Geometry: final body of the model. Coordinates: model frame, mm. A direction names the side the tool comes from. Coordinates: 2 decimals unless noted, no trailing zeros. Use CSV: the item, a comma, the result in double quotes. Start each with the question number.
from build123d import *

# Parameters (mm, degrees)
SKETCH1_R           = 1.5875
BOSS_EXTRUDE1_DEPTH = 1.5748
SKETCH2_W           = 5.842
SKETCH2_H           = 5.842
CUT_EXTRUDE1_DEPTH  = 0.0254
CUT_EXTRUDE2_START  = -1.5748
SKETCH2_2_W         = 5.842
SKETCH2_2_H         = 5.842
CUT_EXTRUDE2_DEPTH  = 0.0254


with BuildPart() as part:
    # Sketch1 → Boss-Extrude1 (new body)
    with BuildSketch(Plane(origin=(0, 0, 0), x_dir=(1, 0, 0), z_dir=(0, 1, 0))):
        Polygon((85.774022, 22.698964), (85.774022, 12.099036), (86.36, 11.557), (86.36, 0), (0, 0), (0, 54.61), (86.36, 54.61), (86.36, 23.241), align=None)
        with Locations((3.175, 51.435)):
            Circle(SKETCH1_R, mode=Mode.SUBTRACT)
        with Locations((3.175, 3.175)):
            Circle(SKETCH1_R, mode=Mode.SUBTRACT)
        with Locations((83.185, 3.175)):
            Circle(SKETCH1_R, mode=Mode.SUBTRACT)
        with Locations((83.185, 51.435)):
            Circle(SKETCH1_R, mode=Mode.SUBTRACT)
    extrude(amount=BOSS_EXTRUDE1_DEPTH)

    # Sketch2 → Cut-Extrude1 (cut)
    with BuildSketch(Plane(origin=(0, 1.5748, 0), x_dir=(1, 0, 0), z_dir=(0, 1, 0))):
        with Locations((3.175, 51.435)):
            Rectangle(SKETCH2_W, SKETCH2_H)
        with Locations((3.175, 3.175)):
            Rectangle(SKETCH2_W, SKETCH2_H)
        with Locations((83.185, 3.175)):
            Rectangle(SKETCH2_W, SKETCH2_H)
        with Locations((83.185, 51.435)):
            Rectangle(SKETCH2_W, SKETCH2_H)
    extrude(amount=-CUT_EXTRUDE1_DEPTH, mode=Mode.SUBTRACT)

    # Sketch2<2> → Cut-Extrude2 (cut)
    with BuildSketch(Plane(origin=(0, 1.5748, 0), x_dir=(1, 0, 0), z_dir=(0, 1, 0)).offset(CUT_EXTRUDE2_START)):
        with Locations((3.175, 51.435)):
            Rectangle(SKETCH2_2_W, SKETCH2_2_H)
        with Locations((3.175, 3.175)):
            Rectangle(SKETCH2_2_W, SKETCH2_2_H)
        with Locations((83.185, 3.175)):
            Rectangle(SKETCH2_2_W, SKETCH2_2_H)
        with Locations((83.185, 51.435)):
            Rectangle(SKETCH2_2_W, SKETCH2_2_H)
    extrude(amount=CUT_EXTRUDE2_DEPTH, mode=Mode.SUBTRACT)


solid = part.part
(1) Mould query, pull axis X, two halves, no side actions, for faces 3 (the face through (84.038, 0.777, -4.514)), 4 (the face through (2.005, 0.777, -4.248)), 5 (the face through (86.36, 1, -6)). Classes: pulls with the +X half, pulls with the -X half, needs draft (parallel to the pull), parting line crosses it, or undercut.
(2) First-contact query: pin 1 (3 mm diameter, centred on x = 2.5, z = -2.5, fed in from -Y); pin 2 (3 mm diameter, centred on x = 82, z = -4.5, fed in from +Y). Flat tips, straight axial feed; report the tip coordinate or a pass-through.
(3) Line query: line 1 (X direction, y = 1.5, z = -16); line 2 (X direction, y = 0.2, z = -50.5). Output: solid intervals per line, ascending. Write a range as from..to.
(4) Access query for faces 1 (the face through (85.774, 1, -17)), 2 (the face through (44, 1, 0)). Directions: +Z, -Z, +X, -X, +Y, -Y. A direction counts if a zero-diameter tool reaches every point of the face in a straight line with its end or side. Return the directions, or none.
Check sheet entries:
1,face 3,"undercut"
1,face 4,"undercut"
1,face 5,"pulls with the +X half"
2,pin 1,"stops at y = 0.03"
2,pin 2,"stops at y = 1.55"
3,line 1,"x = 0..85.77"
3,line 2,"x = 0..1.89, 4.46..81.9, 84.47..86.36"
4,face 1,"+X, +Y, -Y"
4,face 2,"+Z, +X, -X, +Y, -Y"
